Can you work these out from the model? Positions are in its coordinate system, mm. A direction names the side the tool comes from. Coordinates: 2 decimals unless noted, no trailing zeros. Order: outer loops, then holes, each group sorted by start corner. A loop starts at its lowest first (then second) coordinate and runs counter-clockwise, first axis right, second up. Notation, with made-up numbers: (-30, 15) - (7, 15) arc R23 ccw to (7, 27) - close; hole circle Ø3 at (28, 51). An arc over 180 degrees is marked (long way). Use a Markdown table: item, result. Add a question column.
(1) If I drill on L1, parallel to Y at x = -0.25, z = 31.5; L2, parallel to Y at x = 0, z = 8.5; L3, parallel to Z at x = -5.5, y = -3.5, over which ranges is the centre line in solid material (lowest first)? Write a range as [from, to].
(2) For pin 1 Ø8 at (x, z) = (5, 37) entering from +Y; pin 2 Ø10 at (x, z) = (-7, 23) entering from +Y; pin 3 Ø1.5 at (x, z) = (4, 30) entering from -Y, each with a flat end and sliding along its axis, tell me the tip position at first contact or that it passes through.
(3) I want a section at D-D (x = 6). List the corners of the cut face in (y, z) for me.
(4) On a 3-axis mill with a long thin cutter (end or side, diameter ignored), from which of +Z, -Z, +X, -X, +Y, -Y can I reach the whole of each face in a straight line? I mean faces 1 (the flat face through (0, -7.3, 0)), 2 (the flat face through (-5, 2, 25.4)). Say none if no direction works.
(5) We'd pull the mould along X, two halves only. Please class faces 3 (the cylindrical face through (-3.971, -3.045, 37.922)), 4 (the cylindrical face through (3.229, -6.208, 12.522)), 5 (the cylindrical face through (-1.95, -8.79, 25.04)), 6 (the flat face through (4, -4, 50.8)): pulls with the +X half, pulls with the -X half, needs draft (parallel to the pull), parting line crosses it, or undercut.
(6) I want a section at A-A (x = 0). List the corners of the cut face in (y, z) for me, and give its area (3 significant figures).
(7) I want a section at C-C (z = 22). List the corners of the cut face in (x, y) for me.
```python
from build123d import *

# Parameters (mm, degrees)
F0_R          = 9.0043
F1_DEPTH      = 50.8
F2_R          = 5.0038
F3_DEPTH      = 85.09
F3_DEPTH_BACK = 25.4
F4_R          = 6.9977
F5_DEPTH      = 25.4


with BuildPart() as f1:
    # F0 (on Top) → F1 (new body)
    with BuildSketch(Plane.XY):
        Circle(F0_R)
    extrude(amount=F1_DEPTH)

    # F2 (on Top) → F3 (cut, two sides)
    with BuildSketch(Plane.XY) as f3_sk:
        Circle(F2_R)
    extrude(amount=F3_DEPTH, mode=Mode.SUBTRACT)
    extrude(f3_sk.sketch, amount=-F3_DEPTH_BACK, mode=Mode.SUBTRACT)

    # F4 (on Top) → F5 (cut)
    with BuildSketch(Plane.XY):
        Circle(F4_R)
    extrude(amount=F5_DEPTH, mode=Mode.SUBTRACT)


solid = f1.part
```
Answers follow:
| question | item | result |
|---|---|---|
| 1 | L1 | y = [-9, -5], [5, 9] |
| 1 | L2 | y = [-9, -7], [7, 9] |
| 1 | L3 | z = [25.4, 50.8] |
| 2 | pin 1 | stops at y = 8.95 |
| 2 | pin 2 | stops at y = 8.78 |
| 2 | pin 3 | stops at y = -8.4 |
| 3 | outline | (-6.71, 0) - (-3.6, 0) - (-3.6, 25.4) - (3.6, 25.4) - (3.6, 0) - (6.71, 0) - (6.71, 50.8) - (-6.71, 50.8) - close |
| 4 | face 1 | -Z, +X, -X, +Y, -Y |
| 4 | face 2 | -Z |
| 5 | face 3 | undercut |
| 5 | face 4 | undercut |
| 5 | face 5 | parting line crosses it |
| 5 | face 6 | needs draft |
| 6 | outline | (-9, 0) - (-7, 0) - (-7, 25.4) - (-5, 25.4) - (-5, 50.8) - (-9, 50.8) - close; (5, 25.4) - (7, 25.4) - (7, 0) - (9, 0) - (9, 50.8) - (5, 50.8) - close |
| 6 | area | 305 mm² |
| 7 | outline | circle Ø18.01 at (0, 0); hole circle Ø14 at (0, 0) |
